Work out the finished part from the listing and answer in its coordinate system (mm). Face numbers are marked on the shaded views. A direction names the side the tool comes from. Give positions to 0.01 mm unless a question says otherwise; leave off trailing zeros. Loops run counter-clockwise (first coordinate to the right, second up) from the corner with the lowest first, then second, coordinate; pieces in that order, holes last. Notation, with made-up numbers: (5.5, 62.25) -> (39.5, 62.25) arc R34 ccw to (39.5, 98.25) -> close; hole circle Ø8 at (11, 65.25). An arc over 180 degrees is marked (long way). Answer as CSV lines item,"result". Start each with the question number.
1. A tool of negligible diameter and unlimited length cuts with its end or side. For the marked faces 4, 5, 6, 7 and 8, from which of +Z, -Z, +X, -X, +Y, -Y can it reach the whole face along a straight path? Write none if from no direction.
2. Find section A-A, the plane y = -22. Give the vertices of the cut face in (x, z).
3. Find the intervals of material crossed by line 1 along Y through (x, z) = (2.25, 4.5); line 2 along Y through (x, z) = (-2.75, 0); line 3 along Z through (x, y) = (-0.25, -13.5), in increasing order.
4. Determine the mould class of the marked faces 1, 2 and 3 for opening direction Y: +Y half, -Y half, draft (parallel to the pull), parting line (faces both ways), or undercut.
5. Flat-ended cylindrical pins translate along their axes: pin 1 Ø5 at (x, z) = (-9.5, -3.5) entering from +Y; pin 2 Ø3 at (x, y) = (0, -14.59) entering from -Z; pin 3 Ø2.5 at (x, y) = (0.5, -14.5) entering from +Z; pin 4 Ø1.4 at (y, z) = (-14.59, 0) entering from +X. Find the tip coordinate at first contact, or state that the pin passes through.
6. Find section B-B, the plane y = -16.5. Give the vertices of the cut face in (x, z), and give its area (3 significant figures).
7. Find section C-C, the plane y = -7. Give the vertices of the cut face in (x, z).
Autodesk Inventor part; units mm, degrees
ref_plane "YZ Plane" through (0, 0, 0) normal (1, 0, 0) x (0, 1, 0)
ref_plane "XZ Plane" through (0, 0, 0) normal (0, 1, 0) x (-1, 0, 0)
ref_plane "XY Plane" through (0, 0, 0) normal (0, 0, 1) x (1, 0, 0)
sketch "Sketch1" plane through (0, 0, 0) normal (0, 0, 1) x (1, 0, 0)
  line L0 (0, 0) -> (6.0706, 0)
  line L1 (6.0706, 0) -> (6.0706, 12.7)
  line L2 (6.0706, 12.7) -> (4.6228, 12.7)
  line L3 (4.6228, 12.7) -> (4.6228, 15.113)
  line L4 (4.6228, 15.113) -> (6.0706, 15.113)
  line L5 (6.0706, 15.113) -> (6.0706, 18.288)
  line L6 (6.0706, 18.288) -> (0, 18.288)
  line L7 (0, 18.288) -> (0, 0)
  line L8 (0, -29.2334) -> (0, 26.2082)
  line L9 (6.0706, 0) -> (6.0706, 6.35)
  line L10 (6.0706, 0) -> (6.0706, 6.35)
  line L11 (6.0706, 6.35) -> (13.048, -8.6131)
  line L12 (6.0706, 6.35) -> (22.5806, 6.35) construction
  line L13 (13.048, -8.6131) -> (9.873, -8.6131)
  line L14 (9.873, -8.6131) -> (6.0706, 0)
  line L15 (13.048, -8.6131) -> (0, -8.6131)
  line L16 (0, 0) -> (6.0706, 0)
  line L17 (0, -8.6131) -> (12.7, -8.6131)
  line L18 (12.7, -8.6131) -> (12.7, -21.3131)
  line L19 (12.7, -21.3131) -> (0, -21.3131)
  line L20 (0, -21.3131) -> (0, -8.6131)
  line L21 (12.7, -8.6131) -> (12.7, -7.8668)
  dimension "d0" = 6.0706
  dimension "d1" = 12.7
  dimension "d2" = 90
  dimension "d3" = 1.4478
  dimension "d4" = 2.413
  dimension "d5" = 3.175
  dimension "d23" = 16.51
  dimension "d24" = 65
  dimension "d25" = 3.175
  dimension "d83" = 12.7
  dimension "d84" = 12.7
revolve "Revolution1" add sketch "Sketch1" angle 360 about axis through (0, -10, 0) along (0, 1, 0) contours L7 L6 L5 L4 L3 L2 L1 L0 | L0 L14 L15 L8 | L1 L11 L21 L13 L14 | L15 L13 L18 L19 L8
sketch "Sketch12" plane through (0, 18.288, 0) normal (0, 1, 0) x (1, 0, 0)
  point P0 (0, 0)
  point P1 (0, 0)
hole "Hole4" at (0, 18.288, 0) direction (0, -1, 0) diameter 1.5875 depth 32.8676 tip angle 118
sketch "Sketch13" plane through (0, -21.3131, 0) normal (0, -1, 0) x (1, 0, 0)
  circle A0 centre (0, 0) radius 12.7
  point P0 (12.7, 0)
  point P1 (0, -12.7)
  point P2 (-12.7, 0)
  point P3 (0, 12.7)
ref_plane "Work Plane1" through (12.7, -21.3131, 0) normal (1, 0, 0) x (0, 1, 0)
sketch "Sketch14" plane through (12.7, -21.3131, 0) normal (1, 0, 0) x (0, 1, 0)
  line L0 (0, 12.7) -> (0, -12.7)
  line L1 (0, 0) -> (13.4463, 0)
  line L2 (13.4463, 12.7) -> (13.4463, -12.7)
  line L3 (13.4463, 0) -> (6.728, 0)
  point P0 (21.3131, 0)
  dimension "d92" = 6.7183
hole "Hole5" at (12.7, -14.5851, 0) direction (-1, 0, 0) diameter 1.5875 end through all
hole "Hole6" at (12.7, -14.5851, 0) direction (-1, 0, 0) diameter 5.3594 depth 6.35
extrude "Extrusion3" add sketch "Sketch13" along normal blind 6.35
sketch "Sketch16" plane through (0, -27.6631, 0) normal (0, -1, 0) x (1, 0, 0)
  point P0 (0, 0)
hole "Hole8" at (0, -27.6631, 0) direction (0, 1, 0) diameter 4.9784 depth 6.35
pattern_circular "Circular Pattern5" count 4 over 360 about axis through (0, -10, 0) along (0, 1, 0) of "Hole5", "Hole6"
equation "\"d54\" = 55deg"
equation "\"Sketch7_Pitch\" = 0.90714"
equation "\"d72\" = 55deg"
equation "\"Sketch9_Pitch\" = 1.27"
equation "\"d137\" = 55deg"
equation "\"Sketch17_Pitch\" = 1.27"
equation "\"d155\" = 55deg"
equation "\"Sketch19_Pitch\" = 0.90714"
equation "\"d173\" = 55deg"
equation "\"Sketch21_Pitch\" = 0.90714"
equation "\"d191\" = 55deg"
equation "\"Sketch23_Pitch\" = 1.27"
equation "\"d221\" = 55deg"
equation "\"Sketch25_Pitch\" = 0.90714"
equation "\"d239\" = 55deg"
equation "\"Sketch27_Pitch\" = 1.27"
properties part number "piston badflowchannel-1-16in-thread"
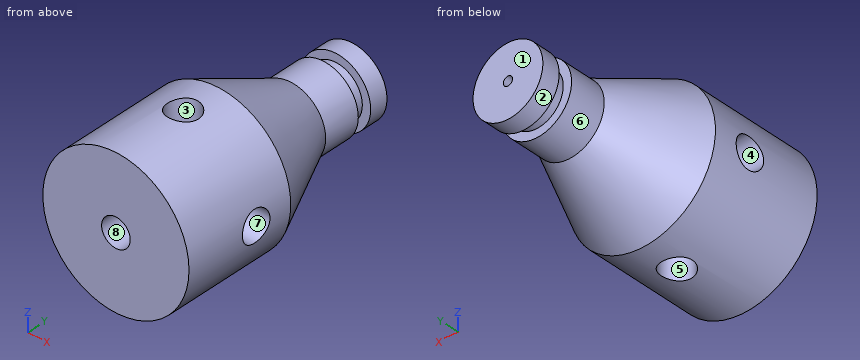
Resolved:
1,face 4,"-X"
1,face 5,"-Z"
1,face 6,"+Y"
1,face 7,"+X"
1,face 8,"-Y"
2,outline,"circle Ø25.4 at (0, 0); hole circle Ø4.98 at (0, 0)"
3,line 1,"y = -27.66 to 12.7, 15.11 to 18.29"
3,line 2,"y = -27.66 to -15.38, -13.79 to 18.29"
3,line 3,"z = -6.35 to -0.75, 0.75 to 6.35"
4,face 1,"+Y half"
4,face 2,"draft"
4,face 3,"undercut"
5,pin 1,"stops at y = 3.02"
5,pin 2,"stops at z = -6.35"
5,pin 3,"stops at z = 6.35"
5,pin 4,"passes through"
6,outline,"(-12.56, -1.87) arc R12.7 ccw to (-1.87, -12.56) -> (-1.87, -6.35) -> (1.87, -6.35) -> (1.87, -12.56) arc R12.7 ccw to (12.56, -1.87) -> (6.35, -1.87) -> (6.35, 1.87) -> (12.56, 1.87) arc R12.7 ccw to (1.87, 12.56) -> (1.87, 6.35) -> (-1.87, 6.35) -> (-1.87, 12.56) arc R12.7 ccw to (-12.56, 1.87) -> (-6.35, 1.87) -> (-6.35, -1.87) -> close"
6,area,"412 mm^2"
7,outline,"circle Ø24.59 at (0, 0); hole circle Ø1.59 at (0, 0)"
